Geometry check sheet. Reference: drawing and pictorial views, mm from the part's lowest x, y, z. A direction names the side the tool comes from. Round coordinates to 2 decimals unless told otherwise and drop trailing zeros. Loops run counter-clockwise (first coordinate to the right, second up) from the corner with the lowest first, then second, coordinate; pieces in that order, holes last. Notation, with made-up numbers: M 48.25,-26 L 89.25,-26 A15 ccw 89.25,0 Z; hole C 19,34 d3. An arc over 180 degrees is marked long. One line per question, with ' | ' between items. Start each with the question number.
(1) Tool access check on the marked faces 1, 2 and 3. Record the directions out of +Z, -Z, +X, -X, +Y, -Y that give a thin tool (end or side, any length) a straight path to the whole face; none if there is none.
(2) Go/stop test with flat-tipped pins: P1, Ø12, axis at y = 42.5, z = 8, coming from the -X side (3 decimals); P2, Ø3, axis at y = 38.5, z = 6, coming from the +X side; P3, Ø6, axis at y = 11, z = 21, coming from the -X side. Record where each tip stops, or that it passes through.
(3) Thickness scan on probe 1 along Y at (x, z) = (15.25, 6); probe 2 along Y at (x, z) = (4.5, 21.5); probe 3 along X at (y, z) = (72, 12.5). Record the ranges inside material, lowest first. Write a range as [from, to].
(4) Section check C-C (y = 15). Record the boundary of the cut face in (x, z) (3 decimals).
(5) Section check D-D (z = 1.75). Record the boundary of the cut face in (x, y), and give its area (3 significant figures).
(6) Section check B-B (x = 12.7). Record the boundary of the cut face in (y, z) (3 decimals).
(7) Section check A-A (z = 12.7). Record the boundary of the cut face in (x, y) (3 decimals), and give its area (3 significant figures).
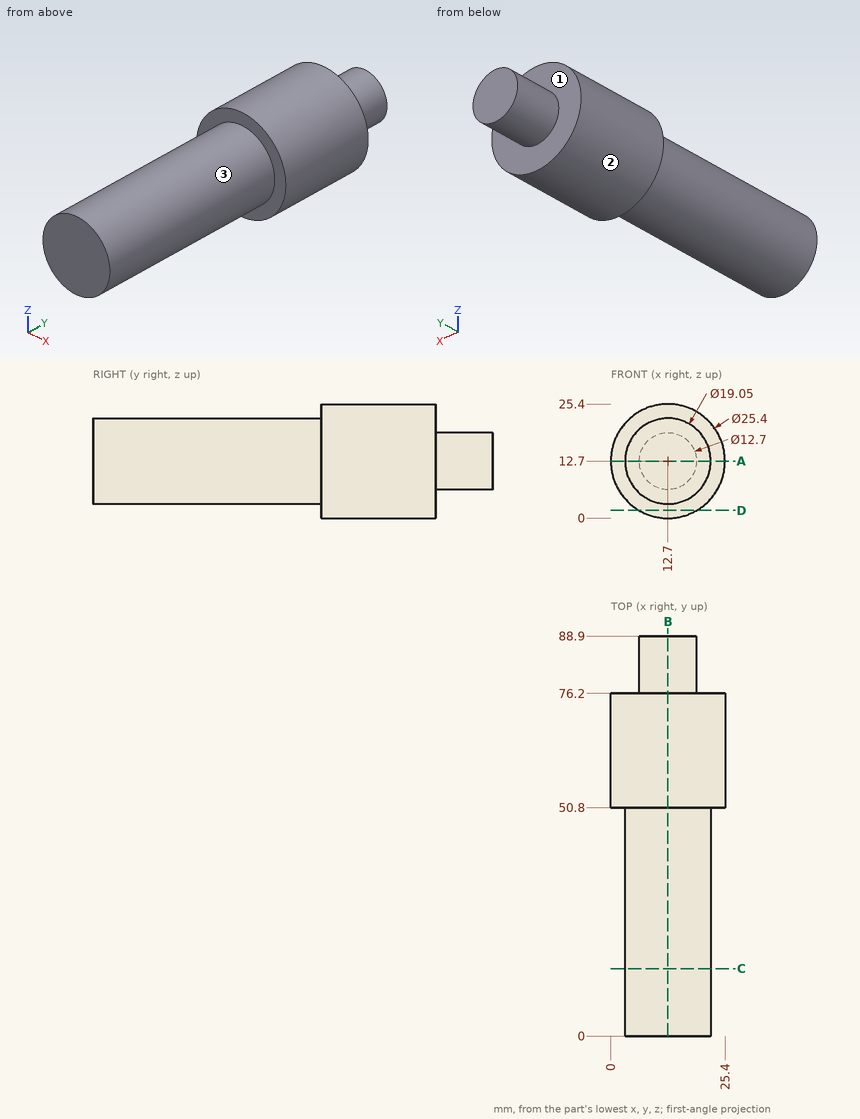
The answers:
1) face 1: +Y | face 2: +Y, -Y | face 3: -Y
2) P1: x = 3.175 | P2: x = 20.68 | P3: x = 4.79
3) probe 1: [0, 76.2] | probe 2: [50.8, 76.2] | probe 3: [0, 25.4]
4) outline: C 12.7,12.7 d19.05
5) outline: M 6.27,50.8 L 19.13,50.8 L 19.13,76.2 L 6.27,76.2 Z | area: 327 mm²
6) outline: M 0,3.175 L 50.8,3.175 L 50.8,0 L 76.2,0 L 76.2,6.35 L 88.9,6.35 L 88.9,19.05 L 76.2,19.05 L 76.2,25.4 L 50.8,25.4 L 50.8,22.225 L 0,22.225 Z
7) outline: M 0,50.8 L 3.175,50.8 L 3.175,0 L 22.225,0 L 22.225,50.8 L 25.4,50.8 L 25.4,76.2 L 19.05,76.2 L 19.05,88.9 L 6.35,88.9 L 6.35,76.2 L 0,76.2 Z | area: 1,770 mm²
